Work out the finished part from the listing and answer in its coordinate system (mm). A direction names the side the tool comes from. Coordinates: 2 decimals unless noted, no trailing zeros. Use a Markdown table: item, result.
from build123d import *

# Parameters (mm, degrees)
BOSS_EXTRUDE1_DEPTH      = 20
BOSS_EXTRUDE2_START      = 40
SKETCH3_R                = 50
BOSS_EXTRUDE2_DEPTH      = 40
BOSS_EXTRUDE3_START      = -40
BOSS_EXTRUDE3_DEPTH      = 40
FILLET1_R                = 25
CIRPATTERN1_COUNT        = 2
CIRPATTERN1_ANGLE        = 90
FILLET1_OF_CIRPATTERN1_R = 25
CIRPATTERN2_COUNT        = 2
FILLET1_OF_CIRPATTERN2_R = 25
BOSS_EXTRUDE4_START      = 20
BOSS_EXTRUDE4_DEPTH      = 20
FILLET2_R                = 8
FILLET3_R                = 8
CUT_EXTRUDE1_DEPTH       = 264.396788984
CIRPATTERN4_COUNT        = 2
CIRPATTERN4_ANGLE        = 180
CIRPATTERN4_COPY_1_DEPTH = 264.396788984
FILLET4_R                = 8
FILLET5_R                = 8
CIRPATTERN6_COUNT        = 2
CIRPATTERN6_ANGLE        = 270
CIRPATTERN6_COPY_1_DEPTH = 264.396788984
FILLET6_R                = 8
FILLET7_R                = 8
CUT_EXTRUDE2_DEPTH       = 8
CIRPATTERN7_COUNT        = 3
CIRPATTERN7_ANGLE        = 180
CUT_EXTRUDE3_DEPTH       = 16
SKETCH21_R               = 7.5
CUT_EXTRUDE4_DEPTH       = 268.16636848
SKETCH22_R               = 10
CUT_EXTRUDE5_DEPTH       = 267.943567929


with BuildPart() as part:
    # Sketch2 → Boss-Extrude1 (new body)
    with BuildSketch(Plane(origin=(0, 0, 0), x_dir=(1, 0, 0), z_dir=(0, 1, 0))):
        with BuildLine():
            Line((-112.127978028, 49.376424233), (0, 31.5))
            ThreePointArc((0, 31.5), (31.5, 0), (0, -31.5))
            Line((0, -31.5), (-112.127978028, -49.376424233))
            ThreePointArc((-112.127978028, -49.376424233), (-170, 0), (-112.127978028, 49.376424233))
        make_face()
    extrude(amount=BOSS_EXTRUDE1_DEPTH)

    # Sketch3 → Boss-Extrude2 (add)
    with BuildSketch(Plane.XZ.offset(BOSS_EXTRUDE2_START)):
        with Locations(Location((-120, 0, 0), (0, 0, 270))):
            Circle(SKETCH3_R)
    extrude(amount=-BOSS_EXTRUDE2_DEPTH)

    # Sketch5 → Boss-Extrude3 (add)
    with BuildSketch(Plane(origin=(0, 20, 0), x_dir=(1, 0, 0), z_dir=(0, 1, 0)).offset(BOSS_EXTRUDE3_START)):
        with BuildLine():
            Line((-130, 114.03716334), (-130, 48.989794856))
            ThreePointArc((-130, 48.989794856), (-121.081407967, 49.9883042), (-112.127978028, 49.376424233))
            Line((-112.127978028, 49.376424233), (-110, 49.03716334))
            Line((-110, 49.03716334), (-110, 114.03716334))
            Line((-110, 114.03716334), (-130, 114.03716334))
        make_face()
    boss_extrude3 = extrude(amount=BOSS_EXTRUDE3_DEPTH)

    # Fillet1
    fillet1_edges = [part.edges().sort_by_distance(p)[0] for p in [
        (-120, 20, -114.03716334),
    ]]
    fillet(fillet1_edges, radius=FILLET1_R)

    # CirPattern1: Boss-Extrude3 ×2 about axis
    cirpattern1_axis = Axis((-120, 0, 0), (0, 1, 0))
    for i in range(1, CIRPATTERN1_COUNT):
        add(boss_extrude3.rotate(cirpattern1_axis, i * CIRPATTERN1_ANGLE / (CIRPATTERN1_COUNT - 1)))

    # Fillet1 of CirPattern1
    fillet1_of_cirpattern1_edges = [part.edges().sort_by_distance(p)[0] for p in [
        (-234.03716334, 20, 0),
    ]]
    fillet(fillet1_of_cirpattern1_edges, radius=FILLET1_OF_CIRPATTERN1_R)

    # CirPattern2: Boss-Extrude3 ×2 about axis
    cirpattern2_axis = Axis((-120, 0, 0), (0, 1, 0))
    for i in range(1, CIRPATTERN2_COUNT):
        add(boss_extrude3.rotate(cirpattern2_axis, i * 360 / CIRPATTERN2_COUNT))

    # Fillet1 of CirPattern2
    fillet1_of_cirpattern2_edges = [part.edges().sort_by_distance(p)[0] for p in [
        (-120, 20, 114.03716334),
    ]]
    fillet(fillet1_of_cirpattern2_edges, radius=FILLET1_OF_CIRPATTERN2_R)

    # Sketch6 → Boss-Extrude4 (add)
    with BuildSketch(Plane.XZ.offset(20).offset(BOSS_EXTRUDE4_START)):
        with BuildLine():
            ThreePointArc((-110, 48.989794856), (-100.123850776, 45.879610853), (-91.100082802, 40.801896842))
            Line((-91.100082802, 40.801896842), (-90, 40.801896842))
            Line((-90, 40.801896842), (-90, 114.03716334))
            Line((-90, 114.03716334), (-110, 114.03716334))
            Line((-110, 114.03716334), (-110, 48.989794856))
        make_face()
        with BuildLine():
            ThreePointArc((-120, 50), (-114.9745519, 49.74680765), (-110, 48.989794856))
            Line((-110, 48.989794856), (-110, 114.03716334))
            Line((-110, 114.03716334), (-120, 114.03716334))
            Line((-120, 114.03716334), (-120, 50))
        make_face()
        with BuildLine():
            Line((-130, 49.03716334), (-127.872021972, 49.376424233))
            ThreePointArc((-127.872021972, 49.376424233), (-123.948340685, 49.843862268), (-120, 50))
            Line((-120, 50), (-120, 114.03716334))
            Line((-120, 114.03716334), (-130, 114.03716334))
            Line((-130, 114.03716334), (-130, 49.03716334))
        make_face()
        with BuildLine():
            Line((-150, 40.801896842), (-148.899917198, 40.801896842))
            ThreePointArc((-148.899917198, 40.801896842), (-138.879208341, 46.298763401), (-127.872021972, 49.376424233))
            Line((-127.872021972, 49.376424233), (-130, 49.03716334))
            Line((-130, 49.03716334), (-130, 114.03716334))
            Line((-130, 114.03716334), (-150, 114.03716334))
            Line((-150, 114.03716334), (-150, 40.801896842))
        make_face()
    boss_extrude4 = extrude(amount=-BOSS_EXTRUDE4_DEPTH)

    # Fillet2
    fillet2_edges = [part.edges().sort_by_distance(p)[0] for p in [
        (-150, -30, 114.03716334),
    ]]
    fillet(fillet2_edges, radius=FILLET2_R)

    # Fillet3
    fillet3_edges = [part.edges().sort_by_distance(p)[0] for p in [
        (-90, -30, 114.03716334),
    ]]
    fillet(fillet3_edges, radius=FILLET3_R)

    # Sketch8 → Cut-Extrude1 (cut, through all)
    with BuildSketch(Plane(origin=(0, -20, 0), x_dir=(1, 0, 0), z_dir=(0, 1, 0))):
        with BuildLine():
            Line((-95, -76.03716334), (-95, -92.03716334))
            ThreePointArc((-95, -92.03716334), (-100, -97.03716334), (-105, -92.03716334))
            Line((-105, -92.03716334), (-105, -76.03716334))
            ThreePointArc((-105, -76.03716334), (-100, -71.03716334), (-95, -76.03716334))
        make_face()
    cut_extrude1 = extrude(amount=-CUT_EXTRUDE1_DEPTH, mode=Mode.SUBTRACT)

    # Mirror1: Cut-Extrude1 across plane
    add(cut_extrude1.mirror(Plane(origin=(-120, 0, 0), x_dir=(0, 0, 1), z_dir=(1, 0, 0))), mode=Mode.SUBTRACT)

    # CirPattern4: Boss-Extrude4, Cut-Extrude1 ×2 about axis
    cirpattern4_axis = Axis((-120, 0, 0), (0, 1, 0))
    add([boss_extrude4.rotate(cirpattern4_axis, i * CIRPATTERN4_ANGLE / (CIRPATTERN4_COUNT - 1)) for i in range(1, CIRPATTERN4_COUNT)])
    add([cut_extrude1.rotate(cirpattern4_axis, i * CIRPATTERN4_ANGLE / (CIRPATTERN4_COUNT - 1)) for i in range(1, CIRPATTERN4_COUNT)], mode=Mode.SUBTRACT)

    # CirPattern4 copy 1 sketch → CirPattern4 copy 1 (cut, through all)
    with BuildSketch(Plane(origin=(0, -20, 0), x_dir=(1, 0, 0), z_dir=(0, 1, 0))):
        with BuildLine():
            Line((-95, 76.03716334), (-95, 92.03716334))
            ThreePointArc((-95, 92.03716334), (-100, 97.03716334), (-105, 92.03716334))
            Line((-105, 92.03716334), (-105, 76.03716334))
            ThreePointArc((-105, 76.03716334), (-100, 71.03716334), (-95, 76.03716334))
        make_face()
    extrude(amount=-CIRPATTERN4_COPY_1_DEPTH, mode=Mode.SUBTRACT)

    # Fillet4
    fillet4_edges = [part.edges().sort_by_distance(p)[0] for p in [
        (-90, -30, -114.03716334),
    ]]
    fillet(fillet4_edges, radius=FILLET4_R)

    # Fillet5
    fillet5_edges = [part.edges().sort_by_distance(p)[0] for p in [
        (-150, -30, -114.03716334),
    ]]
    fillet(fillet5_edges, radius=FILLET5_R)

    # CirPattern6: Boss-Extrude4, Cut-Extrude1 ×2 about axis
    cirpattern6_axis = Axis((-120, 0, 0), (0, 1, 0))
    add([boss_extrude4.rotate(cirpattern6_axis, i * CIRPATTERN6_ANGLE / (CIRPATTERN6_COUNT - 1)) for i in range(1, CIRPATTERN6_COUNT)])
    add([cut_extrude1.rotate(cirpattern6_axis, i * CIRPATTERN6_ANGLE / (CIRPATTERN6_COUNT - 1)) for i in range(1, CIRPATTERN6_COUNT)], mode=Mode.SUBTRACT)

    # CirPattern6 copy 1 sketch → CirPattern6 copy 1 (cut, through all)
    with BuildSketch(Plane(origin=(-120, -20, -120), x_dir=(0, 0, -1), z_dir=(0, 1, 0))):
        with BuildLine():
            Line((-95, 76.03716334), (-95, 92.03716334))
            ThreePointArc((-95, 92.03716334), (-100, 97.03716334), (-105, 92.03716334))
            Line((-105, 92.03716334), (-105, 76.03716334))
            ThreePointArc((-105, 76.03716334), (-100, 71.03716334), (-95, 76.03716334))
        make_face()
    extrude(amount=-CIRPATTERN6_COPY_1_DEPTH, mode=Mode.SUBTRACT)

    # Fillet6
    fillet6_edges = [part.edges().sort_by_distance(p)[0] for p in [
        (-234.03716334, -30, 30),
    ]]
    fillet(fillet6_edges, radius=FILLET6_R)

    # Fillet7
    fillet7_edges = [part.edges().sort_by_distance(p)[0] for p in [
        (-234.03716334, -30, -30),
    ]]
    fillet(fillet7_edges, radius=FILLET7_R)

    # Sketch10 → Revolve1 (revolve)
    with BuildSketch(Plane.XY, mode=Mode.PRIVATE) as revolve1_sk:
        Polygon((31.5, 20), (22.5, 63), (0, 63), (0, 20), align=None)
    revolve(revolve1_sk.sketch.rotate(Axis((0, 0, 0), (0, 1, 0)), 90), axis=Axis((0, 0, 0), (0, 1, 0)))

    # Sketch11 → Cut-Revolve1 (revolve, cut)
    with BuildSketch(Plane.XY, mode=Mode.PRIVATE) as cut_revolve1_sk:
        Polygon((0, 63), (0, 0), (22.5, 0), (12.5, 63), align=None)
    revolve(cut_revolve1_sk.sketch.rotate(Axis((0, 82.375246711, 0), (0, -1, 0)), 90), axis=Axis((0, 82.375246711, 0), (0, -1, 0)), mode=Mode.SUBTRACT)

    # Rib6: read off the stored shape, not the designer's step
    # Rib6: loft between two sections, ruled curve by curve
    rib6_from = [
        Edge.make_line((-69.5, 20, 5), (-31.10064308, 20, 5)),
        Edge.make_line((-31.10064308, 20, -5), (-69.5, 20, -5)),
        Edge.make_line((-69.5, 20, -5), (-69.5, 20, 5)),
        Edge.make_line((-31.10064308, 20, -5), (-31.10064308, 20, 5)),
    ]
    rib6_to = [
        Edge.make_line((-22.5, 63, 5), (-21.937410968, 63, 5)),
        Edge.make_line((-21.937410968, 63, -5), (-22.5, 63, -5)),
        Edge.make_line((-22.5, 63, -5), (-22.5, 63, 5)),
        Edge.make_line((-21.937410968, 63, -5), (-21.937410968, 63, 5)),
    ]
    rib6 = Solid(Shell([*[Face.make_surface_from_curves(rib6_from[k], rib6_to[k]) for k in range(4)], Face(Wire(rib6_from)), Face(Wire(rib6_to))]))
    add(rib6)

    # Sketch15 → Cut-Extrude2 (cut)
    with BuildSketch(Plane(origin=(0, 20, 0), x_dir=(1, 0, 0), z_dir=(0, 1, 0))):
        with BuildLine():
            ThreePointArc((-120, -43), (-77.016651718, 1.196566115), (-122.392205492, 42.933406025))
            ThreePointArc((-122.392205492, 42.933406025), (-132.763210279, 31.338482148), (-121.168286403, 20.967477361))
            ThreePointArc((-121.168286403, 20.967477361), (-99.008132234, 0.584369498), (-120, -21))
            ThreePointArc((-120, -21), (-131, -32), (-120, -43))
        make_face()
    extrude(amount=-CUT_EXTRUDE2_DEPTH, mode=Mode.SUBTRACT)

    # Sketch19 → M12 Tapped Hole1 (revolve, cut)
    with BuildSketch(Plane(origin=(-120, 12, 32), x_dir=(0, 0, 1), z_dir=(1, 0, 0))):
        Polygon((0, 0), (0, 28.064389157), (5.1, 25), (5.1, 0.925), (6.025, 0), align=None)
    m12_tapped_hole1 = revolve(axis=Axis((-120, 18.35, 32), (0, -1, 0)), mode=Mode.SUBTRACT)

    # CirPattern7: M12 Tapped Hole1 ×3 about axis
    cirpattern7_axis = Axis((-120, 0, 0), (0, 1, 0))
    for i in range(1, CIRPATTERN7_COUNT):
        add(m12_tapped_hole1.rotate(cirpattern7_axis, i * CIRPATTERN7_ANGLE / (CIRPATTERN7_COUNT - 1)), mode=Mode.SUBTRACT)

    # Sketch20 → Cut-Extrude3 (cut)
    with BuildSketch(Plane(origin=(0, 20, 0), x_dir=(1, 0, 0), z_dir=(0, 1, 0))):
        with BuildLine():
            ThreePointArc((-133.884701329, 28.8308007), (-151.987608024, -0.890467807), (-132.259263254, -29.55859375))
            ThreePointArc((-132.259263254, -29.55859375), (-127.928821535, -22.33647119), (-120, -19.5))
            ThreePointArc((-120, -19.5), (-100.50755136, 0.54262882), (-121.084837374, 19.469800407))
            ThreePointArc((-121.084837374, 19.469800407), (-129.159180077, 21.860777124), (-133.884701329, 28.8308007))
        make_face()
    extrude(amount=-CUT_EXTRUDE3_DEPTH, mode=Mode.SUBTRACT)

    # Sketch21 → Cut-Extrude4 (cut, through all)
    with BuildSketch(Plane(origin=(0, 20, 0), x_dir=(1, 0, 0), z_dir=(0, 1, 0))):
        with Locations(Location((-151.987608024, -0.890467807, 0), (0, 0, 270))):
            Circle(SKETCH21_R)
    extrude(amount=-CUT_EXTRUDE4_DEPTH, mode=Mode.SUBTRACT)

    # Sketch22 → Cut-Extrude5 (cut, through all)
    with BuildSketch(Plane(origin=(0, 4, 0), x_dir=(1, 0, 0), z_dir=(0, 1, 0))):
        with Locations(Location((-120, 0, 0), (0, 0, 270))):
            Circle(SKETCH22_R)
    extrude(amount=-CUT_EXTRUDE5_DEPTH, mode=Mode.SUBTRACT)


solid = part.part
1. For a pull along Z with two mould halves and no side action, classify faces 1 (the face through (-10, 63, 10)), 2 (the face through (-99.89, -29.86, -97.036)), 3 (the face through (-120.14, 12.48, -106.91)) as +Z half, -Z half, draft (parallel to the pull), parting line (faces both ways), or undercut.
Answers below:
| item | result |
|---|---|
| face 1 | draft |
| face 2 | undercut |
| face 3 | -Z half |
2. Find the intervals of material crossed by probe 1 along X at (y, z) = (-26.5, 0); probe 2 along X at (y, z) = (-27.5, 84); probe 3 along Z at (x, y) = (-114.5, -15), in increasing order.
Answers below:
| item | result |
|---|---|
| probe 1 | -234.04 to -159.43, -144.54 to -130, -110 to -70 |
| probe 2 | -150 to -145, -135 to -105, -95 to -90 |
| probe 3 | -114.04 to -8.35, 8.35 to 114.04 |
3. Section A-A on y = -28 is taken. Give the number of separate pieces and of enclosed holes in the cut face, then the cut area to 3 significant figures.
Answers below:
| item | result |
|---|---|
| separate pieces | 1 |
| enclosed holes | 8 |
| area | 17,900 mm² |
4. For faces 4 (the face through (-201, 0, -10)), 5 (the face through (-150, -30, -73)), 6 (the face through (-99, 12, -10)), 7 (the face through (-140.11, -29.86, -97.036)), determine the directions among +Z, -Z, +X, -X, +Y, -Y from which every point of the face is accessible in a straight line to the end or side of a thin tool.
Answers below:
| item | result |
|---|---|
| face 4 | -Z, -X, +Y |
| face 5 | -Z, -X, +Y, -Y |
| face 6 | +Y |
| face 7 | +Y, -Y |
5. Flat-ended cylindrical pins translate along their axes: P1, Ø6, axis at x = -142.5, z = -93.5, coming from the +Y side; P2, Ø6, axis at x = -88, z = 0, coming from the +Y side; P3, Ø8, axis at y = -29, z = -84, coming from the +X side. Find the tip coordinate at first contact, or state that the pin passes through.
Answers below:
| item | result |
|---|---|
| P1 | y = -20 |
| P2 | y = -14.26 |
| P3 | x = -90 |
